Build history of the part. All positions in model axes, mm. A direction names the side the tool comes from. Round coordinates to 2 decimals unless told otherwise and drop trailing zeros. Order: outer loops, then holes, each group sorted by start corner. A loop starts at its lowest first (then second) coordinate and runs counter-clockwise, first axis right, second up. Notation, with made-up numbers: M -22.5,36 L 9.5,36 A9 ccw 9.5,41 Z; hole C -4.75,-13 d4. An arc over 180 degrees is marked long. One line per item, written item: value. Start each with the question number.
Item 1: Probe L1, parallel to Z at x = -2.45, y = -1.1; L2, parallel to X at y = -0.1, z = -11.25; L3, parallel to Y at x = -0.2, z = -4.5. List the from-to ranges inside material, lowest first.
Item 2: Band-saw the part on A-A, the plane x = 0. Write the cut outline in (y, z) (3 decimals), then the cut area to 3 significant figures.
Item 3: Tool access for faces 1 (the flat face through (1, -1, 0)), 2 (the flat face through (-1.05, 0.61, -0.71)), 3 (the cylindrical face through (-1.5, 0.07, -8.92)): list every direction of +Z, -Z, +X, -X, +Y, -Y with a clear straight run to the whole face (end or side of a thin tool).
Item 4: Band-saw the part on B-B, the plane z = -2.25. Write the cut outline in (x, y) (3 decimals), then the cut area to 3 significant figures.
Item 5: Band-saw the part on D-D, the plane x = 1.9. Write the cut outline in (y, z).
Item 6: Pin check, flat tips, straight feed: pin 1 (1.2 mm diameter, centred on x = -0.5, y = 0, fed in from +Z); pin 2 (1.5 mm diameter, centred on y = -0.5, z = -11, fed in from -X); pin 3 (1.5 mm diameter, centred on x = 0, z = -12, fed in from +Y). Stop position of each tip, or through.
Item 7: Two-plate mould, pull along Y, no slides. Class faces 4 (the flat face through (0, 1.212, -1)), 5 (the flat face through (1.2, -1.2, -3)), 6 (the cylindrical face through (2.6, 0.82, -1.48)): +Y half, -Y half, draft (parallel to the pull), parting line (faces both ways), or undercut.
Item 8: Band-saw the part on C-C, the plane y = 0.85. Write the cut outline in (x, z), then the cut area to 3 significant figures.
Solid Edge part; units mm, degrees
sketch "Sketch1" plane through (0, 0, 0) normal (0, 0, 1) x (1, 0, 0)
  circle A0 centre (0, 0) radius 2.725
extrude "Protrusion1" add sketch "Sketch1" against normal blind 3
sketch "Sketch2" plane through (0, 0, 0) normal (0, 0, 1) x (1, 0, 0)
  line L0 (-0.7, -1.2124) -> (-1.05, -0.6062)
  line L1 (-1.4, 0) -> (-1.05, -0.6062)
  line L2 (-1.4, 0) -> (-1.05, 0.6062)
  line L3 (-0.7, 1.2124) -> (-1.05, 0.6062)
  line L4 (-0.7, 1.2124) -> (0, 1.2124)
  line L5 (0.7, 1.2124) -> (0, 1.2124)
  line L6 (0.7, 1.2124) -> (1.05, 0.6062)
  line L7 (1.4, 0) -> (1.05, 0.6062)
  line L8 (1.4, 0) -> (1.05, -0.6062)
  line L9 (0.7, -1.2124) -> (1.05, -0.6062)
  line L10 (0.7, -1.2124) -> (0, -1.2124)
  line L11 (-0.7, -1.2124) -> (0, -1.2124)
extrude "ExtrudedCutout_1" cut sketch "Sketch2" against normal blind 1.45
sketch "Sketch3" plane through (0, 0, -3) normal (0, 0, -1) x (1, 0, 0)
  circle A0 centre (0, 0) radius 1.5
extrude "ExtrudedProtrusion_2" add sketch "Sketch3" along normal blind 12
cosmetic_thread "Thread1"
properties material "Stainless steel"
Output:
1. L1: z = -3 to 0
1. L2: x = -1.5 to 1.5
1. L3: y = -1.49 to 1.49
2. outline: M -2.725,-3 L -1.5,-3 L -1.5,-15 L 1.5,-15 L 1.5,-3 L 2.725,-3 L 2.725,0 L 1.212,0 L 1.212,-1.45 L -1.212,-1.45 L -1.212,0 L -2.725,0 Z
2. area: 48.8 mm²
3. face 1: +Z, +X, -X, +Y, -Y
3. face 2: +Z
3. face 3: -Z
4. outline: C 0,0 d5.45
4. area: 23.3 mm²
5. outline: M -1.95,-3 L 1.95,-3 L 1.95,0 L -1.95,0 Z
6. pin 1: stops at z = -1.45
6. pin 2: stops at x = -1.5
6. pin 3: stops at y = 1.5
7. face 4: undercut
7. face 5: draft
7. face 6: parting line
8. outline: M -2.59,-3 L -1.24,-3 L -1.24,-15 L 1.24,-15 L 1.24,-3 L 2.59,-3 L 2.59,0 L 0.91,0 L 0.91,-1.45 L -0.91,-1.45 L -0.91,0 L -2.59,0 Z
8. area: 42.6 mm²
